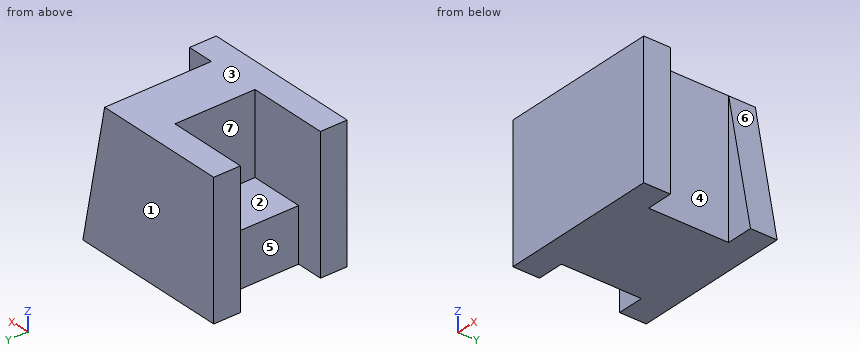
```python
from build123d import *

# Parameters (mm, degrees)
BOSS_EXTRUDE1_DEPTH = 25
SKETCH2_W           = 10
SKETCH2_H           = 15
BOSS_EXTRUDE2_DEPTH = 10
SKETCH3_W           = 25
SKETCH3_H           = 5
BOSS_EXTRUDE3_DEPTH = 5
CUT_EXTRUDE1_DEPTH  = 5


with BuildPart() as part:
    # Sketch1 → Boss-Extrude1 (new body)
    with BuildSketch(Plane.XY):
        Polygon((0, 0), (25, 0), (25, 25), (0, 25), (0, 20), (15, 20), (15, 5), (0, 5), align=None)
    extrude(amount=BOSS_EXTRUDE1_DEPTH)

    # Sketch2 → Boss-Extrude2 (add)
    with BuildSketch(Plane.ZY.offset(-15)):
        with Locations((5, 12.5)):
            Rectangle(SKETCH2_W, SKETCH2_H)
    extrude(amount=BOSS_EXTRUDE2_DEPTH)

    # Sketch3 → Boss-Extrude3 (add)
    with BuildSketch(Plane(origin=(25, 0, 0), x_dir=(0, 0, -1), z_dir=(1, 0, 0))):
        with Locations((-12.5, 22.5)):
            Rectangle(SKETCH3_W, SKETCH3_H)
        with Locations((-12.5, 2.5)):
            Rectangle(SKETCH3_W, SKETCH3_H)
    extrude(amount=BOSS_EXTRUDE3_DEPTH)

    # Sketch4 → Cut-Extrude1 (cut)
    with BuildSketch(Plane(origin=(0, 25, 0), x_dir=(1, 0, 0), z_dir=(0, 1, 0))):
        Polygon((25, -25), (30, 0), (30, -25), align=None)
    extrude(amount=-CUT_EXTRUDE1_DEPTH, mode=Mode.SUBTRACT)


solid = part.part
```
Could you check a few things on this model? Use its own coordinates, in mm. Face numbers are marked on the shaded views. A direction names the side the tool comes from. Round coordinates to 2 decimals unless told otherwise and drop trailing zeros. Loops run counter-clockwise (first coordinate to the right, second up) from the corner with the lowest first, then second, coordinate; pieces in that order, holes last. Notation, with made-up numbers: M -15,77.5 L 35,77.5 A14 cw 35,84.5 Z; hole C 76,-5 d11. An arc over 180 degrees is marked long. Put each result on its own line as item: value.
Q1. For pin 1 (10 mm diameter, centred on y = 14.5, z = 4, fed in from +X); pin 2 (11 mm diameter, centred on y = 11, z = 5.5, fed in from -X); pin 3 (10 mm diameter, centred on y = 20.5, z = 6, fed in from +X), each with a flat end and sliding along its axis, tell me the tip position at first contact or that it passes through.
Check result:
pin 1: x = 25
pin 2: x = 5
pin 3: x = 29.8
Q2. Imagine slicing it at A-A (z = 19.5). Write out the boundary of the cut face in (x, y), then the cut area to 4 significant figures.
Check result:
outline: M 0,0 L 30,0 L 30,5 L 25,5 L 25,20 L 26.1,20 L 26.1,25 L 0,25 L 0,20 L 15,20 L 15,5 L 0,5 Z
area: 430.5 mm2
Q3. Thinking about a two-plate mould opening in Y: for the marked faces 1, 2 and 3, which applies, released by +Y, released by -Y, zero draft, split by the parting line, or undercut?
Check result:
face 1: released by +Y
face 2: undercut
face 3: zero draft
Q4. On a 3-axis mill with a long thin cutter (end or side, diameter ignored), from which of +Z, -Z, +X, -X, +Y, -Y can I reach the whole of each face in a straight line? I mean the marked faces 4, 5, 6 and 7. Say none if no direction works.
Check result:
face 4: +Z, -Z, +X
face 5: +Z, -Z, -X
face 6: +Z, +X, +Y
face 7: +Z, -X
Q5. Imagine slicing it at B-B (x = 8.75). Write out the boundary of the cut face in (y, z).
Check result:
outline: M 0,0 L 25,0 L 25,25 L 20,25 L 20,10 L 5,10 L 5,25 L 0,25 Z
Q6. I need wall thicknesses on probe 1 along Y at (x, z) = (10.5, 17); probe 2 along X at (y, z) = (7.75, 22.5); probe 3 along Z at (x, y) = (11.5, 13.25). Which ranges of each line are inside material? Lowest first, please.
Check result:
probe 1: 0 to 5, 20 to 25
probe 2: 15 to 25
probe 3: 0 to 10
Q7. Imagine slicing it at D-D (z = 3). Write out the boundary of the cut face in (x, y), then the cut area to 3 significant figures.
Check result:
outline: M 0,0 L 30,0 L 30,5 L 25,5 L 25,20 L 29.4,20 L 29.4,25 L 0,25 L 0,20 L 5,20 L 5,5 L 0,5 Z
area: 597 mm2
Q8. Imagine slicing it at C-C (y = 23). Write out the boundary of the cut face in (x, z).
Check result:
outline: M 0,0 L 30,0 L 25,25 L 0,25 Z
